Read the model definition and answer for the solid it produces. Units are mm, in the model's axes. Give positions to 0.01 mm unless a question says otherwise; leave off trailing zeros. Order: outer loops, then holes, each group sorted by start corner. A loop starts at its lowest first (then second) coordinate and runs counter-clockwise, first axis right, second up. Notation, with made-up numbers: (-12.5, -24.75) -> (10.5, -24.75) arc R27 cw to (10.5, -0.75) -> close; hole circle Ø10 at (-23, 28). An arc over 180 degrees is marked (long way). Use one line per item in the form item = value.
```python
from build123d import *

# Parameters (mm, degrees)
SKETCH1_W           = 494
SKETCH1_H           = 15
BOSS_EXTRUDE1_DEPTH = 10
SKETCH3_R           = 5
CUT_EXTRUDE1_DEPTH  = 10
SKETCH4_R           = 5
CUT_EXTRUDE2_DEPTH  = 10


with BuildPart() as part:
    # Sketch1 → Boss-Extrude1 (new body)
    with BuildSketch(Plane.YZ):
        with Locations((247, 7.5)):
            Rectangle(SKETCH1_W, SKETCH1_H)
    extrude(amount=BOSS_EXTRUDE1_DEPTH)

    # Sketch3 → Cut-Extrude1 (cut)
    with BuildSketch(Plane.YZ):
        with Locations(Location((7.5, 7.5, 0), (0, 0, 270))):
            Circle(SKETCH3_R)
    extrude(amount=CUT_EXTRUDE1_DEPTH, mode=Mode.SUBTRACT)

    # Sketch4 → Cut-Extrude2 (cut)
    with BuildSketch(Plane.YZ.offset(10)):
        with Locations(Location((486.5, 7.5, 0), (0, 0, 270))):
            Circle(SKETCH4_R)
    extrude(amount=-CUT_EXTRUDE2_DEPTH, mode=Mode.SUBTRACT)


solid = part.part
```
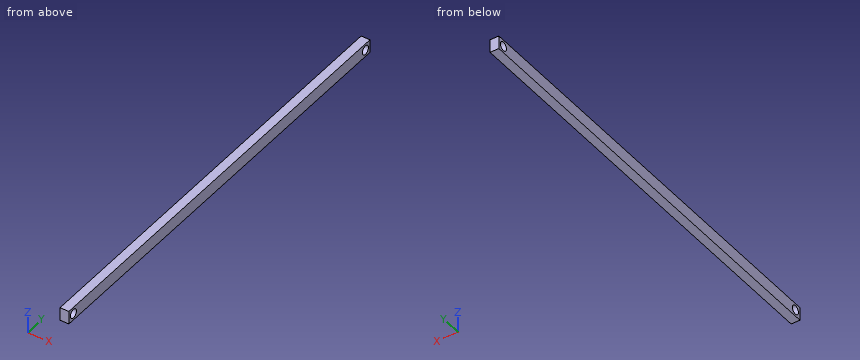
Item 1: The part is cut by section B-B on y = 7.5. Give the vertices of the cut face in (x, z), and give its area (3 significant figures).
Checks:
outline = (0, 0) -> (10, 0) -> (10, 2.5) -> (0, 2.5) -> close; (0, 12.5) -> (10, 12.5) -> (10, 15) -> (0, 15) -> close
area = 50.0 mm²
Item 2: The part is cut by section A-A on z = 7.5. Give the vertices of the cut face in (x, y), and give its area (3 significant figures).
Checks:
outline = (0, 0) -> (10, 0) -> (10, 2.5) -> (0, 2.5) -> close; (0, 12.5) -> (10, 12.5) -> (10, 481.5) -> (0, 481.5) -> close; (0, 491.5) -> (10, 491.5) -> (10, 494) -> (0, 494) -> close
area = 4,740 mm²
Item 3: Given pin 1 Ø6 at (x, y) = (3.5, 406) entering from -Z, flat-ended and moving along its own axis, determine where the tip first touches the part or whether it passes through.
Checks:
pin_1 = 0
Item 4: The part is cut by section C-C on x = 1.5. Give the vertices of the cut face in (y, z), and give its area (3 significant figures).
Checks:
outline = (0, 0) -> (494, 0) -> (494, 15) -> (0, 15) -> close; hole circle Ø10 at (7.5, 7.5); hole circle Ø10 at (486.5, 7.5)
area = 7,250 mm²
Item 5: Straight lines are drawn through the part: L1, parallel to Y at x = 2.5, z = 7.25; L2, parallel to Y at x = 2.5, z = 5.75; L3, parallel to Z at x = 4.5, y = 486.5. For each, find the intervals that lie inside material, in ascending order. Write a range as from..to.
Checks:
L1 = 0..2.51, 12.49..481.51, 491.49..494
L2 = 0..2.82, 12.18..481.82, 491.18..494
L3 = 0..2.5, 12.5..15
